Input: part model. Units: mm. Frame: model coordinates. Face numbers are marked on the shaded views. A direction names the side the tool comes from. Give positions to 0.01 mm unless a question says otherwise; leave off trailing zeros. Loops run counter-clockwise (first coordinate to the right, second up) from the corner with the lowest first, then second, coordinate; pieces in that order, holes last.
Autodesk Inventor part; units mm, degrees
ref_plane "YZ Plane" through (0, 0, 0) normal (1, 0, 0) x (0, 1, 0)
ref_plane "XZ Plane" through (0, 0, 0) normal (0, 1, 0) x (-1, 0, 0)
ref_plane "XY Plane" through (0, 0, 0) normal (0, 0, 1) x (1, 0, 0)
sketch "Boceto1" plane through (0, 0, 0) normal (0, 1, 0) x (-1, 0, 0)
  line L0 (0, 0) -> (26, 0)
  line L1 (26, 0) -> (26, -45)
  line L2 (26, -45) -> (0, -45)
  line L3 (0, -45) -> (0, 0)
  dimension "d0" = 26
  dimension "d1" = 45
extrude "Extrusión1" add sketch "Boceto1" along normal blind 5
sketch "Boceto2" plane through (0, 5, 0) normal (0, 1, 0) x (1, 0, 0)
  line L0 (-26, 0) -> (0, 0)
  line L1 (0, 0) -> (-5, 0)
  line L2 (0, 45) -> (-26, 45)
  line L3 (-26, 45) -> (-21, 45)
  line L4 (0, 45) -> (0, 40)
  line L5 (0, 0) -> (0, 45)
  line L6 (0, 0) -> (0, 5)
  line L7 (-26, 45) -> (-26, 0)
  circle A0 centre (-21, 40) radius 2.5
  circle A1 centre (-5, 5) radius 2.5
  dimension "d4" = 5
  dimension "d6" = 5
  dimension "d7" = 5
  dimension "d9" = 5
  dimension "d10" = 5
extrude "Extrusión2" cut sketch "Boceto2" against normal blind 5 contours A0 | A1
sketch "Boceto3" plane through (0, 5, 0) normal (0, 1, 0) x (1, 0, 0)
  line L0 (0, 0) -> (0, 45)
  line L1 (0, 45) -> (0, 37.5)
  line L2 (0, 45) -> (0, 30)
  line L3 (0, 0) -> (0, 15)
  line L4 (-5.5, 15) -> (-20.5, 15)
  line L5 (-20.5, 15) -> (-20.5, 30)
  line L6 (-20.5, 30) -> (-5.5, 30)
  line L7 (-5.5, 30) -> (-5.5, 15)
extrude "Extrusión3" add sketch "Boceto3" along normal blind 40
sketch "Boceto4" plane through (0, 45, 0) normal (0, 1, 0) x (1, 0, 0)
  line L0 (-5.5, 30) -> (-20.5, 30)
  line L1 (-20.5, 30) -> (-20.5, 15)
  line L2 (-20.5, 30) -> (-20.5, 15)
  line L3 (-5.5, 15) -> (-5.5, 30)
  circle A0 centre (-13, 22.5) radius 25
  point P0 (0, 0)
extrude "Extrusión4" add sketch "Boceto4" along normal blind 10
fillet "Empalme1" radius 4 12 edges at (-13, 45, -30) (-5.5, 25, -30) (-5.5, 45, -22.5) (-5.5, 25, -15) (-20.5, 25, -30) (-20.5, 25, -15) (-13, 45, -15) (-20.5, 45, -22.5) (-20.5, 5, -22.5) (-13, 5, -15) (-13, 5, -30) (-5.5, 5, -22.5)
sketch "Boceto6" plane through (-13, 55, -22.5) normal (0, 1, 0) x (1, 0, 0)
  circle A0 centre (0, -20) radius 3
  line L0 (0, 0) -> (31.4027, 0) construction
  line L1 (0, 0) -> (28.2843, 0) construction
  circle A1 centre (14.1421, 14.1421) radius 3
  circle A2 centre (-14.1421, 14.1421) radius 3
  circle A3 centre (-14.1421, -14.1421) radius 3
  circle A4 centre (14.1421, -14.1421) radius 3
  point P0 (13, -22.5)
  dimension "d27" = 6
  dimension "d32" = 6
  dimension "d33" = 6
  dimension "d34" = 6
  dimension "d35" = 6
extrude "Extrusión5" cut sketch "Boceto6" against normal blind 10
properties part number "Flange"
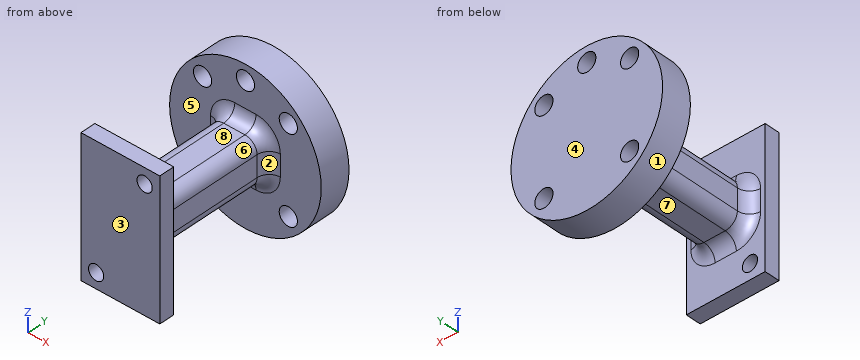
(1) Cut plane A-A (x = -13). Return the cut outline in (y, z).
Values follow:
outline: (0, -45) - (5, -45) - (5, -34) arc R4 cw to (9, -30) - (41, -30) arc R4 cw to (45, -34) - (45, -47.5) - (55, -47.5) - (55, -5.5) - (45, -5.5) - (45, -11) arc R4 cw to (41, -15) - (9, -15) arc R4 cw to (5, -11) - (5, 0) - (0, 0) - close; (45, 0.5) - (55, 0.5) - (55, 2.5) - (45, 2.5) - close
(2) Ray query, probe 1 along Y at (x, z) = (-11, -44); probe 2 along Z at (x, y) = (-5, 3.1); probe 3 along Z at (x, y) = (-21, 3.3). Return the intervals inside material, ascending.
Values follow:
probe 1: y = 0 to 5, 45 to 55
probe 2: z = -45 to -7.5, -2.5 to 0
probe 3: z = -45 to -42.5, -37.5 to 0
(3) Mould query, pull axis Y, two halves, no side actions, for the marked faces 1, 2, 3 and 4. Classes: +Y half, -Y half, draft (parallel to the pull), parting line (faces both ways), or undercut.
Values follow:
face 1: draft
face 2: undercut
face 3: -Y half
face 4: +Y half
(4) Pin query (flat end, axial travel): pin 1 Ø1 at (y, z) = (22.5, -32) entering from +X; pin 2 Ø5.5 at (x, z) = (-27.14, -8.36) entering from +Y; pin 3 Ø10 at (y, z) = (30.5, -20) entering from -X; pin 4 Ø6 at (y, z) = (16.5, -23) entering from +X. Return the tip coordinate at first contact, or that it passes through.
Values follow:
pin 1: passes through
pin 2: stops at y = 5
pin 3: stops at x = -20.5
pin 4: stops at x = -5.5
(5) Cut plane B-B (z = -10). Return the cut outline in (x, y), and give its area (3 significant figures).
Values follow:
outline: (-34.65, 45) - (-29.65, 45) - (-29.65, 55) - (-34.65, 55) - close; (-26, 0) - (0, 0) - (0, 5) - (-26, 5) - close; (-24.63, 45) - (-1.37, 45) - (-1.37, 55) - (-24.63, 55) - close; (3.65, 45) - (8.65, 45) - (8.65, 55) - (3.65, 55) - close
area: 463 mm2
(6) Reachability of the marked faces 5, 6, 7 and 8 from +Z, -Z, +X, -X, +Y, -Y: full face, straight path, thin tool, end or side. Return the list, or none.
Values follow:
face 5: none
face 6: +Z, +X
face 7: -Z, +X, -X
face 8: +Z, +X, -X
(7) Cut plane D-D (x = -28). Return the cut outline in (y, z).
Values follow:
outline: (45, -42.5) - (55, -42.5) - (55, -39.52) - (45, -39.52) - close; (45, -33.77) - (55, -33.77) - (55, -11.23) - (45, -11.23) - close; (45, -5.48) - (55, -5.48) - (55, -2.5) - (45, -2.5) - close
(8) Cut plane C-C (y = 39.5). Return the cut outline in (x, z), and give its area (3 significant figures).
Values follow:
outline: (-20.5, -26) arc R4 ccw to (-16.5, -30) - (-9.5, -30) arc R4 ccw to (-5.5, -26) - (-5.5, -19) arc R4 ccw to (-9.5, -15) - (-16.5, -15) arc R4 ccw to (-20.5, -19) - close
area: 211 mm2
